Here's how the part is built. I have some questions about the finished solid (model axes, mm). Face numbers are marked on the shaded views. A direction names the side the tool comes from. Give positions to 0.01 mm unless a question says otherwise; leave off trailing zeros. Order: outer loops, then holes, each group sorted by start corner. A loop starts at its lowest first (then second) coordinate and runs counter-clockwise, first axis right, second up.
from build123d import *

# Parameters (mm, degrees)
SKETCH1_W                      = 20
SKETCH1_H                      = 65
BOSS_EXTRUDE1_DEPTH            = 19
CBORE_FOR_M5_SHCS1_D           = 5.8
CBORE_FOR_M5_SHCS1_CBORE_D     = 10
CBORE_FOR_M5_SHCS1_CBORE_DEPTH = 5
FILLET1_R                      = 2


with BuildPart() as part:
    # Sketch1 → Boss-Extrude1 (new body)
    with BuildSketch(Plane.XY):
        Rectangle(SKETCH1_W, SKETCH1_H)
    extrude(amount=BOSS_EXTRUDE1_DEPTH)

    # CBORE for M5 SHCS1 (through all)
    with Locations(Plane.XY.offset(19)):
        with Locations((0, -2.5), (0, -22.5)):
            CounterBoreHole(CBORE_FOR_M5_SHCS1_D / 2, CBORE_FOR_M5_SHCS1_CBORE_D / 2, CBORE_FOR_M5_SHCS1_CBORE_DEPTH)

    # Fillet1
    fillet1_edges = [part.edges().sort_by_distance(p)[0] for p in [
        (10, -32.5, 9.5),
        (-10, -32.5, 9.5),
        (-10, 32.5, 9.5),
        (10, 32.5, 9.5),
    ]]
    fillet(fillet1_edges, radius=FILLET1_R)


solid = part.part
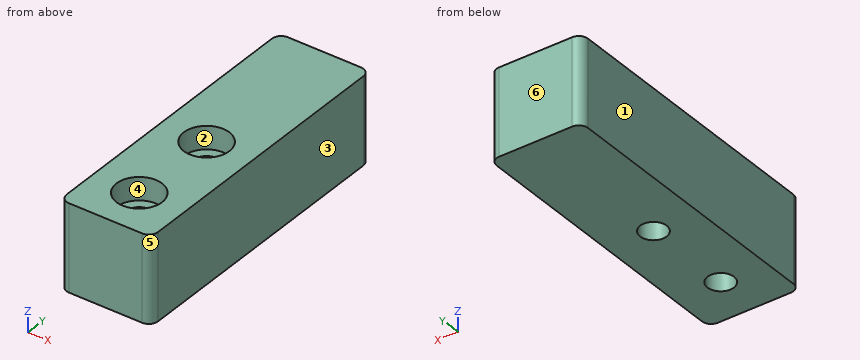
Q1. I'm going to push a flat-ended pin straight in: P1, Ø8, axis at x = 0, y = -22.5, coming from the +Z side. Where does the tip first touch, or does it pass through?
Filled sheet:
P1: stops at z = 14
Q2. Thinking about a two-plate mould opening in Y: for the marked faces 3, 4, 5 and 6, which applies, released by +Y, released by -Y, zero draft, split by the parting line, or undercut?
Filled sheet:
face 3: zero draft
face 4: undercut
face 5: released by -Y
face 6: released by +Y
Q3. If we section it at A-A on y = -22.5: List the corners of the cut face in (x, z) for me.
Filled sheet:
outline: (-10, 0) - (-2.9, 0) - (-2.9, 14) - (-5, 14) - (-5, 19) - (-10, 19) - close; (2.9, 0) - (10, 0) - (10, 19) - (5, 19) - (5, 14) - (2.9, 14) - close
Q4. If we section it at D-D on z = 15: List the corners of the cut face in (x, y) for me.
Filled sheet:
outline: (-10, -30.5) arc R2 ccw to (-8, -32.5) - (8, -32.5) arc R2 ccw to (10, -30.5) - (10, 30.5) arc R2 ccw to (8, 32.5) - (-8, 32.5) arc R2 ccw to (-10, 30.5) - close; hole circle Ø10 at (0, -22.5); hole circle Ø10 at (0, -2.5)
Q5. I need wall thicknesses on L1, parallel to Y at x = 0, z = 17.6; L2, parallel to Y at x = 0, z = 8.25; L3, parallel to X at y = -2, z = 6. Which ranges of each line are inside material? Lowest first, please.
Filled sheet:
L1: y = -32.5 to -27.5, -17.5 to -7.5, 2.5 to 32.5
L2: y = -32.5 to -25.4, -19.6 to -5.4, 0.4 to 32.5
L3: x = -10 to -2.86, 2.86 to 10
Q6. For the marked faces 1 and 2, which set-ups out of +Z, -Z, +X, -X, +Y, -Y let a thin tool reach every point of the face, with its end or its side?
Filled sheet:
face 1: +Z, -Z, -X, +Y, -Y
face 2: +Z
Q7. If we section it at B-B on x = 0: List the corners of the cut face in (y, z) for me.
Filled sheet:
outline: (-32.5, 0) - (-25.4, 0) - (-25.4, 14) - (-27.5, 14) - (-27.5, 19) - (-32.5, 19) - close; (-19.6, 0) - (-5.4, 0) - (-5.4, 14) - (-7.5, 14) - (-7.5, 19) - (-17.5, 19) - (-17.5, 14) - (-19.6, 14) - close; (0.4, 0) - (32.5, 0) - (32.5, 19) - (2.5, 19) - (2.5, 14) - (0.4, 14) - close
Q8. If we section it at C-C on z = 11.25: List the corners of the cut face in (x, y) for me.
Filled sheet:
outline: (-10, -30.5) arc R2 ccw to (-8, -32.5) - (8, -32.5) arc R2 ccw to (10, -30.5) - (10, 30.5) arc R2 ccw to (8, 32.5) - (-8, 32.5) arc R2 ccw to (-10, 30.5) - close; hole circle Ø5.8 at (0, -22.5); hole circle Ø5.8 at (0, -2.5)
